Check sheet for the drawn part. Datum: minimum x, y, z corner. Units: mm. A direction names the side the tool comes from. Round coordinates to 2 decimals unless told otherwise and drop trailing zeros. Order: outer loops, then holes, each group sorted by start corner. A loop starts at its lowest first (then second) coordinate and runs counter-clockwise, first axis right, second up. Notation, with made-up numbers: (-31, 31) -> (-14, 31) arc R6 ccw to (-14, 37) -> close; hole circle Ø2 at (69.5, -36.5). An arc over 180 degrees is marked (long way). Answer as a JSON object with one key per item and string values. Group by question number.
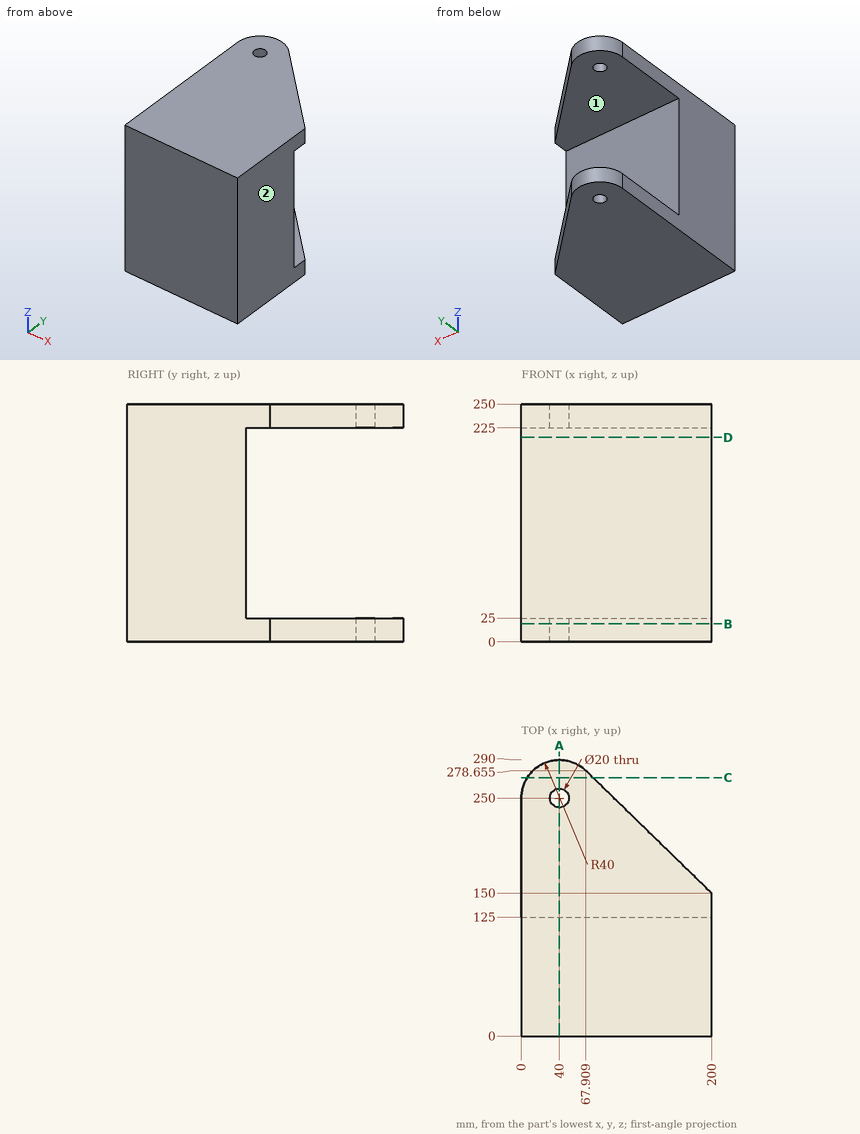
Item 1: Sectioned sample at B-B, the plane z = 19. Enter the section's corners in (x, y) (1 decimal).
Item 2: Depth check by flat-ended pin: pin 1 Ø3 at (x, z) = (154, 133.5) entering from +Y. Enter the tip coordinate at first touch or a pass-through.
Item 3: Set-up check for the marked faces 1 and 2: record each of +Z, -Z, +X, -X, +Y, -Y from which the full face is reachable in a straight line by a thin tool's end or side.
Item 4: Sectioned sample at A-A, the plane x = 40. Enter the section's corners in (y, z).
Item 5: Sectioned sample at D-D, the plane z = 215. Enter the section's corners in (x, y), then the cut area to 3 significant figures.
Item 6: Thickness scan on L1, parallel to Y at x = 40, z = 10; L2, parallel to Z at x = 165, y = 133.5; L3, parallel to Y at x = 152, z = 137. Record the ranges inside material, lowest first.
Item 7: Sectioned sample at C-C, the plane y = 271.5. Enter the section's corners in (x, z) (1 decimal), then the cut area to 3 significant figures.
Result:
{
 "1": {"outline": "(0, 0) -> (200, 0) -> (200, 150) -> (67.9, 278.7) arc R40 ccw to (0, 250) -> close; hole circle Ø20 at (40, 250)"},
 "2": {"pin 1": "stops at y = 125"},
 "3": {"face 1": "+X, -X, +Y", "face 2": "+Z, -Z, +X, +Y, -Y"},
 "4": {"outline": "(0, 0) -> (240, 0) -> (240, 25) -> (125, 25) -> (125, 225) -> (240, 225) -> (240, 250) -> (0, 250) -> close; (260, 0) -> (290, 0) -> (290, 25) -> (260, 25) -> close; (260, 225) -> (290, 225) -> (290, 250) -> (260, 250) -> close"},
 "5": {"outline": "(0, 0) -> (200, 0) -> (200, 125) -> (0, 125) -> close", "area": "25,000 mm2"},
 "6": {"L1": "y = 0 to 240, 260 to 290", "L2": "z = 0 to 25, 225 to 250", "L3": "y = 0 to 125"},
 "7": {"outline": "(6.3, 0) -> (75.3, 0) -> (75.3, 25) -> (6.3, 25) -> close; (6.3, 225) -> (75.3, 225) -> (75.3, 250) -> (6.3, 250) -> close", "area": "3,450 mm2"}
}
